from build123d import *

# Parameters (mm, degrees)
SKETCH1_W           = 50.8
SKETCH1_H           = 25.4
SKETCH1_W_2         = 47.625
SKETCH1_H_2         = 22.225
BOSS_EXTRUDE1_DEPTH = 660.4
SKETCH2_R           = 2.4892
CUT_EXTRUDE1_DEPTH  = 51.8


with BuildPart() as part:
    # Sketch1 → Boss-Extrude1 (new body)
    with BuildSketch(Plane.XY):
        with Locations((25.4, 12.7)):
            Rectangle(SKETCH1_W, SKETCH1_H)
        with Locations((25.4, 12.7)):
            Rectangle(SKETCH1_W_2, SKETCH1_H_2, mode=Mode.SUBTRACT)
    extrude(amount=BOSS_EXTRUDE1_DEPTH)

    # Sketch2 → Cut-Extrude1 (cut, through all)
    with BuildSketch(Plane.ZY):
        with Locations((12.7, 12.7)):
            Circle(SKETCH2_R)
        with Locations((25.4, 12.7)):
            Circle(SKETCH2_R)
        with Locations((38.1, 12.7)):
            Circle(SKETCH2_R)
        with Locations((50.8, 12.7)):
            Circle(SKETCH2_R)
        with Locations((63.5, 12.7)):
            Circle(SKETCH2_R)
        with Locations((76.2, 12.7)):
            Circle(SKETCH2_R)
        with Locations((88.9, 12.7)):
            Circle(SKETCH2_R)
        with Locations((101.6, 12.7)):
            Circle(SKETCH2_R)
        with Locations((114.3, 12.7)):
            Circle(SKETCH2_R)
        with Locations((127, 12.7)):
            Circle(SKETCH2_R)
        with Locations((139.7, 12.7)):
            Circle(SKETCH2_R)
        with Locations((152.4, 12.7)):
            Circle(SKETCH2_R)
        with Locations((165.1, 12.7)):
            Circle(SKETCH2_R)
        with Locations((177.8, 12.7)):
            Circle(SKETCH2_R)
        with Locations((190.5, 12.7)):
            Circle(SKETCH2_R)
        with Locations((203.2, 12.7)):
            Circle(SKETCH2_R)
        with Locations((215.9, 12.7)):
            Circle(SKETCH2_R)
        with Locations((228.6, 12.7)):
            Circle(SKETCH2_R)
        with Locations((241.3, 12.7)):
            Circle(SKETCH2_R)
        with Locations((254, 12.7)):
            Circle(SKETCH2_R)
        with Locations((266.7, 12.7)):
            Circle(SKETCH2_R)
        with Locations((279.4, 12.7)):
            Circle(SKETCH2_R)
        with Locations((292.1, 12.7)):
            Circle(SKETCH2_R)
        with Locations((304.8, 12.7)):
            Circle(SKETCH2_R)
        with Locations((317.5, 12.7)):
            Circle(SKETCH2_R)
        with Locations((330.2, 12.7)):
            Circle(SKETCH2_R)
        with Locations((342.9, 12.7)):
            Circle(SKETCH2_R)
        with Locations((355.6, 12.7)):
            Circle(SKETCH2_R)
        with Locations((368.3, 12.7)):
            Circle(SKETCH2_R)
        with Locations((381, 12.7)):
            Circle(SKETCH2_R)
        with Locations((393.7, 12.7)):
            Circle(SKETCH2_R)
        with Locations((406.4, 12.7)):
            Circle(SKETCH2_R)
        with Locations((419.1, 12.7)):
            Circle(SKETCH2_R)
        with Locations((431.8, 12.7)):
            Circle(SKETCH2_R)
        with Locations((444.5, 12.7)):
            Circle(SKETCH2_R)
        with Locations((457.2, 12.7)):
            Circle(SKETCH2_R)
        with Locations((469.9, 12.7)):
            Circle(SKETCH2_R)
        with Locations((482.6, 12.7)):
            Circle(SKETCH2_R)
        with Locations((495.3, 12.7)):
            Circle(SKETCH2_R)
        with Locations((508, 12.7)):
            Circle(SKETCH2_R)
        with Locations((520.7, 12.7)):
            Circle(SKETCH2_R)
        with Locations((533.4, 12.7)):
            Circle(SKETCH2_R)
        with Locations((546.1, 12.7)):
            Circle(SKETCH2_R)
        with Locations((558.8, 12.7)):
            Circle(SKETCH2_R)
        with Locations((571.5, 12.7)):
            Circle(SKETCH2_R)
        with Locations((584.2, 12.7)):
            Circle(SKETCH2_R)
        with Locations((596.9, 12.7)):
            Circle(SKETCH2_R)
        with Locations((609.6, 12.7)):
            Circle(SKETCH2_R)
        with Locations((622.3, 12.7)):
            Circle(SKETCH2_R)
        with Locations((635, 12.7)):
            Circle(SKETCH2_R)
        with Locations((647.7, 12.7)):
            Circle(SKETCH2_R)
    extrude(amount=-CUT_EXTRUDE1_DEPTH, mode=Mode.SUBTRACT)


solid = part.part
Source: CAD feature listing. Evaluate the final solid. Frame: model axes, mm. A direction names the side the tool comes from. Give positions to 0.01 mm unless a question says otherwise; leave off trailing zeros. Write each loop counter-clockwise with the first axis right and the second up, starting at its lowest first coordinate (ties: lowest second). Pieces come first, ordered by that corner, then holes. Notation, with made-up numbers: M -6,75 L 42,75 A27 ccw 42,112 Z; hole C 6,79 d4. An arc over 180 degrees is marked long. Return JSON: item names as keys, results as strings. Group by question number.
1) First-contact query: pin 1 Ø3 at (y, z) = (12.7, 25.4) entering from -X. Flat tip, straight axial feed; report the tip coordinate or a pass-through.
2) Ray query, L1, parallel to X at y = 10.25, z = 129; L2, parallel to Y at x = 1, z = 228; L3, parallel to Y at x = 32, z = 413. Return the intervals inside material, ascending.
3) Cut plane A-A, the plane x = 27. Output: boundary loops of the cut face in (y, z).
4) Draft query along Y for faces 3 (the face through (1.587, 13, 326)), 4 (the face through (25, 0, 326)), 5 (the face through (0, 13, 326)). Return one class per face: released by +Y, released by -Y, zero draft, split by the parting line, or undercut.
5) Set-up query: faces 1 (the face through (23, 1, 0)), 2 (the face through (49.212, 13, 326)). Return all of +Z, -Z, +X, -X, +Y, -Y with unobstructed straight access to the full face (end or side cutting, diameter ignored); none if empty.
Data:
{
 "1": {"pin 1": "passes through"},
 "2": {"L1": "x = 0 to 1.59, 49.21 to 50.8", "L2": "y = 0 to 10.28, 15.12 to 25.4", "L3": "y = 0 to 1.59, 23.81 to 25.4"},
 "3": {"outline": "M 0,0 L 1.59,0 L 1.59,660.4 L 0,660.4 Z; M 23.81,0 L 25.4,0 L 25.4,660.4 L 23.81,660.4 Z"},
 "4": {"face 3": "undercut", "face 4": "released by -Y", "face 5": "zero draft"},
 "5": {"face 1": "-Z, +X, -X, +Y, -Y", "face 2": "+Z, -Z"}
}
